Geometry check sheet. Reference: the model listing, model coordinates, mm. A direction names the side the tool comes from. Round coordinates to 2 decimals unless told otherwise and drop trailing zeros. Loops run counter-clockwise (first coordinate to the right, second up) from the corner with the lowest first, then second, coordinate; pieces in that order, holes last. Notation, with made-up numbers: M -16.5,-12 L 25.5,-12 A16 ccw 25.5,8 Z; hole C -30,61 d3. An arc over 180 degrees is marked long. Write item = value, one per line.
from build123d import *

# Parameters (mm, degrees)
SKETCH1_R               = 2.4
BOSS_EXTRUDE1_DEPTH     = 20
SKETCH2_R               = 1.195
CUT_EXTRUDE1_DEPTH      = 10
SKETCH4_R               = 4.85
BOSS_EXTRUDE2_DEPTH     = 2.54
BOSS_EXTRUDE3_START     = -3.35
SKETCH6_R               = 4.85
BOSS_EXTRUDE3_DEPTH     = 3.35
CUT_EXTRUDE3_DEPTH      = 3.3
CUT_EXTRUDE3_DEPTH_BACK = 3.302
SKETCH5_R               = 3.25


with BuildPart() as part:
    # Sketch1 → Boss-Extrude1 (new body)
    with BuildSketch(Plane(origin=(0, 0, 0), x_dir=(1, 0, 0), z_dir=(0, 1, 0))):
        with Locations(Location((0, 0, 0), (0, 0, 270))):
            Circle(SKETCH1_R)
    extrude(amount=BOSS_EXTRUDE1_DEPTH)

    # Sketch2 → Cut-Extrude1 (cut)
    with BuildSketch(Plane.XZ):
        with Locations(Location((0, 0, 0), (0, 0, 270))):
            Circle(SKETCH2_R)
    extrude(amount=-CUT_EXTRUDE1_DEPTH, mode=Mode.SUBTRACT)

    # Sketch4 → Boss-Extrude2 (add)
    with BuildSketch(Plane(origin=(0, 20, 0), x_dir=(1, 0, 0), z_dir=(0, 1, 0))):
        with Locations(Location((0, 0, 0), (0, 0, 270))):
            Circle(SKETCH4_R)
    extrude(amount=BOSS_EXTRUDE2_DEPTH)

    # Sketch6 → Boss-Extrude3 (add)
    with BuildSketch(Plane(origin=(0, 22.54, 0), x_dir=(1, 0, 0), z_dir=(0, 1, 0)).offset(BOSS_EXTRUDE3_START)):
        with Locations(Location((0, 0, 0), (0, 0, 270))):
            Circle(SKETCH6_R)
    extrude(amount=BOSS_EXTRUDE3_DEPTH)

    # Sketch5 → Cut-Extrude3 (cut, two sides: drawn at the far end of the back side and taken through both)
    with BuildSketch(Plane.XY.offset(-CUT_EXTRUDE3_DEPTH_BACK)):
        with Locations((0, 22.54)):
            Circle(SKETCH5_R)
    extrude(amount=CUT_EXTRUDE3_DEPTH + CUT_EXTRUDE3_DEPTH_BACK, mode=Mode.SUBTRACT)


solid = part.part
(1) Tool access check on faces 1 (the flat face through (4, 22.54, 0)), 2 (the cylindrical face through (2.024, 9.461, 1.29)), 3 (the flat face through (0, 21, -3.302)). Record the directions out of +Z, -Z, +X, -X, +Y, -Y that give a thin tool (end or side, any length) a straight path to the whole face; none if there is none.
Result set:
face_1 = +Z, -Z, +X, -X, +Y
face_2 = -Y
face_3 = +Y
(2) Depth check by flat-ended pin: pin 1 Ø2 at (x, y) = (1, 14) entering from -Z; pin 2 Ø2 at (x, z) = (1, 3) entering from +Y; pin 3 Ø1 at (x, y) = (-1.5, 21) entering from -Z; pin 4 Ø5 at (y, z) = (9.5, -1) entering from -X. Enter the tip coordinate at first touch or a pass-through.
Result set:
pin_1 = -2.4
pin_2 = 22.54
pin_3 = -4.75
pin_4 = -2.4
(3) Material ranges on line 1 along X through (y, z) = (5, 0) (3 decimals); line 2 along X through (y, z) = (21.5, -1.5); line 3 along Y through (x, z) = (3.5, -2.5), recorded low to high. Write a range as from..to.
Result set:
line_1 = -2.4..-1.195, 1.195..2.4
line_2 = -4.61..-3.08, 3.08..4.61
line_3 = 19.19..22.54
(4) Sectioned sample at B-B on x = 0. Record the cut outline in (y, z) (3 decimals).
Result set:
outline = M 0,-2.4 L 19.19,-2.4 L 19.19,-4.85 L 22.54,-4.85 L 22.54,-3.302 L 19.29,-3.302 L 19.29,3.3 L 22.54,3.3 L 22.54,4.85 L 19.19,4.85 L 19.19,2.4 L 0,2.4 L 0,1.195 L 10,1.195 L 10,-1.195 L 0,-1.195 Z
(5) Release check for a two-part mould opening along X. For faces 4 (the flat face through (0, 21, 3.3)), 5 (the cylindrical face through (1.457, 20.842, 4.626)), 6 (the flat face through (1, 0, -1)) record: released by +X, released by -X, zero draft, split by the parting line, or undercut.
Result set:
face_4 = undercut
face_5 = split by the parting line
face_6 = zero draft
(6) Sectioned sample at C-C on y = 20.5. Record the cut outline in (x, z), then the cut area to 3 significant figures.
Result set:
outline = C 0,0 d9.7; hole M -2.53,-3.3 L 2.53,-3.3 L 2.53,3.3 L -2.53,3.3 Z
area = 40.5 mm2
(7) Sectioned sample at A-A on z = 0. Record the cut outline in (x, y) (3 decimals), then the cut area to 3 significant figures.
Result set:
outline = M -4.85,19.19 L -2.4,19.19 L -2.4,0 L -1.195,0 L -1.195,10 L 1.195,10 L 1.195,0 L 2.4,0 L 2.4,19.19 L 4.85,19.19 L 4.85,22.54 L 3.25,22.54 A3.25 cw -3.25,22.54 L -4.85,22.54 Z
area = 84.1 mm2
(8) Sectioned sample at D-D on y = 17.25. Record the cut outline in (x, z), then the cut area to 3 significant figures.
Result set:
outline = C 0,0 d4.8
area = 18.1 mm2
